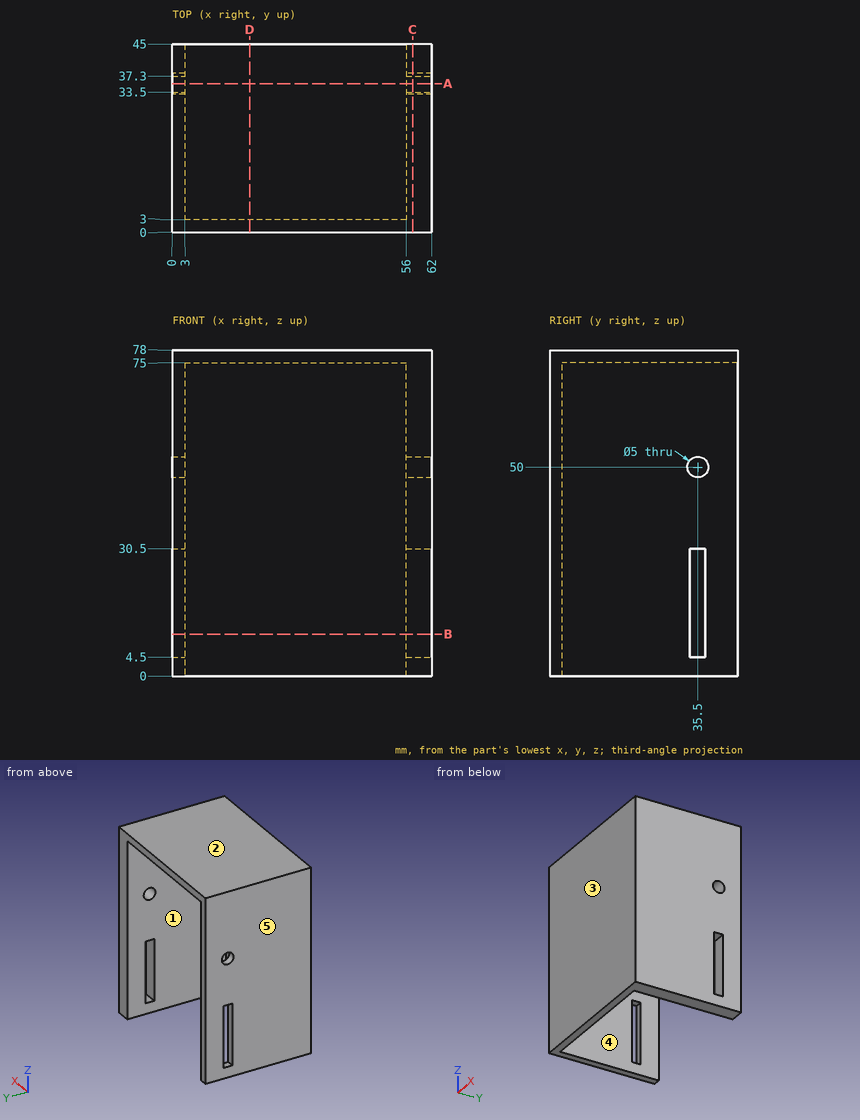
Part print with two shaded views. Sizes in mm from the minimum x, y, z corner. A direction names the side the tool comes from. Round coordinates to 2 decimals unless told otherwise and drop trailing zeros. Write each loop counter-clockwise with the first axis right and the second up, starting at its lowest first coordinate (ties: lowest second). Pieces come first, ordered by that corner, then holes. Notation, with made-up numbers: (37.25, 59) -> (81.25, 59) arc R22 cw to (81.25, 96) -> close; hole circle Ø11 at (77.25, -5.75). An arc over 180 degrees is marked (long way). Use one line per item in the form item = value.
Q1. Band-saw the part on A-A, the plane y = 35.5. Write the cut outline in (x, z), then the cut area to 3 significant figures.
Conclusion:
outline = (0, 0) -> (3, 0) -> (3, 4.5) -> (0, 4.5) -> close; (0, 30.5) -> (3, 30.5) -> (3, 47.5) -> (0, 47.5) -> close; (0, 52.5) -> (3, 52.5) -> (3, 75) -> (56, 75) -> (56, 52.5) -> (62, 52.5) -> (62, 78) -> (0, 78) -> close; (56, 0) -> (62, 0) -> (62, 4.5) -> (56, 4.5) -> close; (56, 30.5) -> (62, 30.5) -> (62, 47.5) -> (56, 47.5) -> close
area = 582 mm²
Q2. Drop flat-ended pins along their axis: P1, Ø21, axis at x = 30.5, y = 16.5, coming from the -Z side; P2, Ø3.5, axis at x = 2, z = 15, coming from the -Y side; P3, Ø12, axis at x = 47, z = 43.5, coming from the +Y side; P4, Ø3, axis at y = 35.5, z = 50, coming from the -X side. Give the stop position or say it passes through.
Conclusion:
P1 = 75
P2 = 0
P3 = 3
P4 = through
Q3. Band-saw the part on D-D, the plane x = 18.5. Write the cut outline in (y, z).
Conclusion:
outline = (0, 0) -> (3, 0) -> (3, 75) -> (45, 75) -> (45, 78) -> (0, 78) -> close
Q4. Tool access for the marked faces 1 and 2: list every direction of +Z, -Z, +X, -X, +Y, -Y with a clear straight run to the whole face (end or side of a thin tool).
Conclusion:
face_1 = -Z, +Y
face_2 = +Z, +X, -X, +Y, -Y
Q5. Two-plate mould, pull along X, no slides. Class the marked faces 3, 4 and 5: released by +X, released by -X, zero draft, split by the parting line, or undercut.
Conclusion:
face_3 = zero draft
face_4 = undercut
face_5 = released by -X
Q6. Drill centre lines: L1, parallel to Y at x = 59, z = 50; L2, parallel to X at y = 33, z = 18.5; L3, parallel to Z at x = 2, y = 35. Where is each one in solid material? Low to high.
Conclusion:
L1 = 0 to 33, 38 to 45
L2 = 0 to 3, 56 to 62
L3 = 0 to 4.5, 30.5 to 47.55, 52.45 to 78
Q7. Band-saw the part on B-B, the plane z = 10. Write the cut outline in (x, y), then the cut area to 3 significant figures.
Conclusion:
outline = (0, 0) -> (62, 0) -> (62, 33.5) -> (56, 33.5) -> (56, 3) -> (3, 3) -> (3, 33.5) -> (0, 33.5) -> close; (0, 37.3) -> (3, 37.3) -> (3, 45) -> (0, 45) -> close; (56, 37.3) -> (62, 37.3) -> (62, 45) -> (56, 45) -> close
area = 530 mm²
Q8. Band-saw the part on C-C, the plane x = 57.5. Write the cut outline in (y, z).
Conclusion:
outline = (0, 0) -> (45, 0) -> (45, 78) -> (0, 78) -> close; hole circle Ø5 at (35.5, 50); hole (33.5, 4.5) -> (37.3, 4.5) -> (37.3, 30.5) -> (33.5, 30.5) -> close
